```python
from build123d import *

# Parameters (mm, degrees)
SKETCH_1_W          = 35
SKETCH_1_H          = 9
EXTRUDE_1_DEPTH     = 5
SKETCH_2_R          = 1.25
SKETCH_2_R_2        = 0.725
SKETCH_2_R_3        = 1.27
SKETCH_2_R_4        = 0.4
CUT_EXTRUDE_1_DEPTH = 5


with BuildPart() as part:
    # 草图1 → 凸台-拉伸1 (new body)
    with BuildSketch(Plane(origin=(0, 0, 0), x_dir=(1, 0, 0), z_dir=(0, 1, 0))):
        Rectangle(SKETCH_1_W, SKETCH_1_H)
    extrude(amount=EXTRUDE_1_DEPTH)

    # 草图2 → 切除-拉伸1 (cut)
    with BuildSketch(Plane(origin=(0, 5, 0), x_dir=(1, 0, 0), z_dir=(0, 1, 0))):
        with Locations(Location((-16, 3, 0), (0, 0, 270))):
            Circle(SKETCH_2_R)
        with Locations(Location((-13.090909091, 3, 0), (0, 0, 270))):
            Circle(SKETCH_2_R)
        with Locations(Location((-10.181818182, 3, 0), (0, 0, 270))):
            Circle(SKETCH_2_R)
        with Locations(Location((-7.272727273, 3, 0), (0, 0, 270))):
            Circle(SKETCH_2_R)
        with Locations(Location((-4.363636364, 3, 0), (0, 0, 270))):
            Circle(SKETCH_2_R)
        with Locations(Location((-1.454545455, 3, 0), (0, 0, 270))):
            Circle(SKETCH_2_R)
        with Locations(Location((1.454545455, 3, 0), (0, 0, 270))):
            Circle(SKETCH_2_R)
        with Locations(Location((4.363636364, 3, 0), (0, 0, 270))):
            Circle(SKETCH_2_R)
        with Locations(Location((7.272727273, 3, 0), (0, 0, 270))):
            Circle(SKETCH_2_R)
        with Locations(Location((10.181818182, 3, 0), (0, 0, 270))):
            Circle(SKETCH_2_R)
        with Locations(Location((13.090909091, 3, 0), (0, 0, 270))):
            Circle(SKETCH_2_R)
        with Locations(Location((16, 3, 0), (0, 0, 270))):
            Circle(SKETCH_2_R)
        with Locations(Location((-16, 0.4, 0), (0, 0, 270))):
            Circle(SKETCH_2_R_2)
        with Locations(Location((-13.090909091, 0.4, 0), (0, 0, 270))):
            Circle(SKETCH_2_R_2)
        with Locations(Location((-10.181818182, 0.4, 0), (0, 0, 270))):
            Circle(SKETCH_2_R_2)
        with Locations(Location((-7.272727273, 0.4, 0), (0, 0, 270))):
            Circle(SKETCH_2_R_2)
        with Locations(Location((-4.363636364, 0.4, 0), (0, 0, 270))):
            Circle(SKETCH_2_R_2)
        with Locations(Location((-1.454545455, 0.4, 0), (0, 0, 270))):
            Circle(SKETCH_2_R_2)
        with Locations(Location((1.454545455, 0.4, 0), (0, 0, 270))):
            Circle(SKETCH_2_R_2)
        with Locations(Location((4.363636364, 0.4, 0), (0, 0, 270))):
            Circle(SKETCH_2_R_2)
        with Locations(Location((7.272727273, 0.4, 0), (0, 0, 270))):
            Circle(SKETCH_2_R_2)
        with Locations(Location((10.181818182, 0.4, 0), (0, 0, 270))):
            Circle(SKETCH_2_R_2)
        with Locations(Location((13.090909091, 0.4, 0), (0, 0, 270))):
            Circle(SKETCH_2_R_2)
        with Locations(Location((16, 0.4, 0), (0, 0, 270))):
            Circle(SKETCH_2_R_2)
        with Locations(Location((-16, -2.2, 0), (0, 0, 270))):
            Circle(SKETCH_2_R_3)
        with Locations(Location((-13.090909091, -2.2, 0), (0, 0, 270))):
            Circle(SKETCH_2_R_3)
        with Locations(Location((-10.181818182, -2.2, 0), (0, 0, 270))):
            Circle(SKETCH_2_R_3)
        with Locations(Location((-7.272727273, -2.2, 0), (0, 0, 270))):
            Circle(SKETCH_2_R_3)
        with Locations(Location((-4.363636364, -2.2, 0), (0, 0, 270))):
            Circle(SKETCH_2_R_3)
        with Locations(Location((-1.454545455, -2.2, 0), (0, 0, 270))):
            Circle(SKETCH_2_R_3)
        with Locations(Location((1.454545455, -2.2, 0), (0, 0, 270))):
            Circle(SKETCH_2_R_3)
        with Locations(Location((4.363636364, -2.2, 0), (0, 0, 270))):
            Circle(SKETCH_2_R_3)
        with Locations(Location((7.272727273, -2.2, 0), (0, 0, 270))):
            Circle(SKETCH_2_R_3)
        with Locations(Location((10.181818182, -2.2, 0), (0, 0, 270))):
            Circle(SKETCH_2_R_3)
        with Locations(Location((13.090909091, -2.2, 0), (0, 0, 270))):
            Circle(SKETCH_2_R_3)
        with Locations(Location((16, -2.2, 0), (0, 0, 270))):
            Circle(SKETCH_2_R_3)
        with Locations(Location((-16.7, -3.9, 0), (0, 0, 270))):
            Circle(SKETCH_2_R_4)
        with Locations(Location((-14.939473684, -3.9, 0), (0, 0, 270))):
            Circle(SKETCH_2_R_4)
        with Locations(Location((-13.178947368, -3.9, 0), (0, 0, 270))):
            Circle(SKETCH_2_R_4)
        with Locations(Location((-11.418421053, -3.9, 0), (0, 0, 270))):
            Circle(SKETCH_2_R_4)
        with Locations(Location((-9.657894737, -3.9, 0), (0, 0, 270))):
            Circle(SKETCH_2_R_4)
        with Locations(Location((-7.897368421, -3.9, 0), (0, 0, 270))):
            Circle(SKETCH_2_R_4)
        with Locations(Location((-6.136842105, -3.9, 0), (0, 0, 270))):
            Circle(SKETCH_2_R_4)
        with Locations(Location((-4.376315789, -3.9, 0), (0, 0, 270))):
            Circle(SKETCH_2_R_4)
        with Locations(Location((-2.615789474, -3.9, 0), (0, 0, 270))):
            Circle(SKETCH_2_R_4)
        with Locations(Location((-0.855263158, -3.9, 0), (0, 0, 270))):
            Circle(SKETCH_2_R_4)
        with Locations(Location((0.905263158, -3.9, 0), (0, 0, 270))):
            Circle(SKETCH_2_R_4)
        with Locations(Location((2.665789474, -3.9, 0), (0, 0, 270))):
            Circle(SKETCH_2_R_4)
        with Locations(Location((4.426315789, -3.9, 0), (0, 0, 270))):
            Circle(SKETCH_2_R_4)
        with Locations(Location((6.186842105, -3.9, 0), (0, 0, 270))):
            Circle(SKETCH_2_R_4)
        with Locations(Location((7.947368421, -3.9, 0), (0, 0, 270))):
            Circle(SKETCH_2_R_4)
        with Locations(Location((9.707894737, -3.9, 0), (0, 0, 270))):
            Circle(SKETCH_2_R_4)
        with Locations(Location((11.468421053, -3.9, 0), (0, 0, 270))):
            Circle(SKETCH_2_R_4)
        with Locations(Location((13.228947368, -3.9, 0), (0, 0, 270))):
            Circle(SKETCH_2_R_4)
        with Locations(Location((14.989473684, -3.9, 0), (0, 0, 270))):
            Circle(SKETCH_2_R_4)
        with Locations(Location((16.75, -3.9, 0), (0, 0, 270))):
            Circle(SKETCH_2_R_4)
    extrude(amount=-CUT_EXTRUDE_1_DEPTH, mode=Mode.SUBTRACT)


solid = part.part
```
Here's how the part is built. I have some questions about the finished solid (model axes, mm). Give positions to 0.01 mm unless a question says otherwise; leave off trailing zeros. Order: outer loops, then holes, each group sorted by start corner. A loop starts at its lowest first (then second) coordinate and runs counter-clockwise, first axis right, second up. Notation, with made-up numbers: M 41,24 L 49,24 A23 ccw 49,45 Z; hole C 64,-34 d5. An arc over 180 degrees is marked long. Use a Markdown table: item, result. Add a question column.
1. Suppose I cut it at B-B (z = -0.4). Give the number of separate pieces and of enclosed holes in the cut face, and give its area (3 significant figures).
2. If we mould it in two halves opening along X, with no side actions, what happens to faces 1 (the flat face through (17.5, 2, 0)), 2 (the flat face through (0, 2, -4.5)), 3 (the cylindrical face through (-2.694, 2.535, 1.925))? For each: +X half, -X half, draft (parallel to the pull), parting line (faces both ways), or undercut.
3. Suppose I cut it at A-A (x = 16). List the corners of the cut face in (y, z) for me (3 decimals).
4. I need wall thicknesses on probe 1 along Z at (x, y) = (11, 1.45); probe 2 along Z at (x, y) = (-10, 4); probe 3 along Z at (x, y) = (-2, 0.5). Which ranges of each line are inside material? Lowest first, please. Write a range as from..to.
Results list:
| question | item | result |
|---|---|---|
| 1 | separate pieces | 13 |
| 1 | enclosed holes | 0 |
| 1 | area | 88.0 mm² |
| 2 | face 1 | +X half |
| 2 | face 2 | draft |
| 2 | face 3 | undercut |
| 3 | outline | M 0,-4.5 L 5,-4.5 L 5,-4.25 L 0,-4.25 Z; M 0,-1.75 L 5,-1.75 L 5,-1.125 L 0,-1.125 Z; M 0,0.325 L 5,0.325 L 5,0.93 L 0,0.93 Z; M 0,3.47 L 5,3.47 L 5,4.5 L 0,4.5 Z |
| 4 | probe 1 | z = -4.5..-3.95, -2.05..1.23, 3.17..4.5 |
| 4 | probe 2 | z = -4.5..-4.24, -1.76..-1.1, 0.3..0.94, 3.46..3.69, 4.11..4.5 |
| 4 | probe 3 | z = -4.5..-4.12, -1.88..-0.88, 0.08..1.05, 3.35..4.5 |
